Read the model definition and answer for the solid it produces. Units are mm, in the model's axes. Face numbers are marked on the shaded views. Coordinates: 2 decimals unless noted, no trailing zeros. Order: outer loops, then holes, each group sorted by start corner. A loop starts at its lowest first (then second) coordinate and runs counter-clockwise, first axis right, second up. Notation, with made-up numbers: M 20.5,1.5 L 29.5,1.5 A17 cw 29.5,17.5 Z; hole C -2,-31 d8. An arc over 180 degrees is marked long. Use a Markdown table: item, result. Add a question column.
1) Find the intervals of material crossed by probe 1 along X at (y, z) = (145, 0); probe 2 along X at (y, z) = (59.5, -2), in increasing order. Write a range as [from, to].
2) The mould has two halves that part along Y. Classify the marked faces 1 and 2: released by +Y, released by -Y, zero draft, split by the parting line, or undercut.
3) Each of these flat-tipped pins is pushed along its axis until it touches: pin 1 Ø8 at (y, z) = (69, 6) entering from +X; pin 2 Ø3.5 at (x, y) = (-145, 145) entering from +Z; pin 3 Ø10 at (x, y) = (65, 15.5) entering from +Z; pin 4 Ø8 at (x, y) = (68.5, -74) entering from -Z. Where does it stop, or does it pass through?
4) Find section A-A on x = 79. Write down the section's boundary in (y, z), plus the area to 3 significant figures.
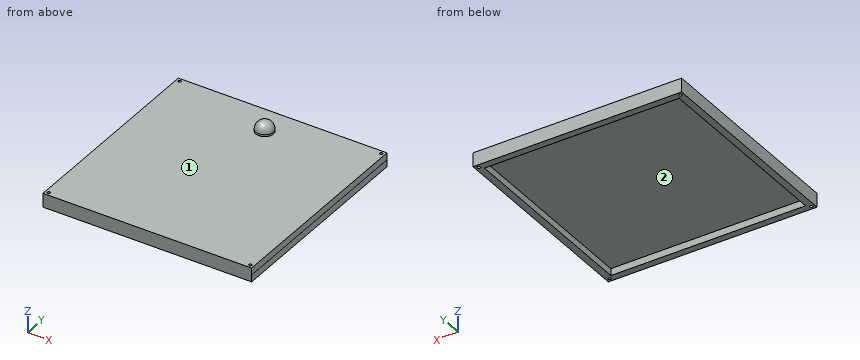
Autodesk Inventor part; units mm, degrees
ref_plane "YZ Plane" through (0, 0, 0) normal (1, 0, 0) x (0, 1, 0)
ref_plane "XZ Plane" through (0, 0, 0) normal (0, 1, 0) x (-1, 0, 0)
ref_plane "XY Plane" through (0, 0, 0) normal (0, 0, 1) x (1, 0, 0)
sketch "Sketch1" plane through (0, 0, 0) normal (0, 0, 1) x (1, 0, 0)
  line L0 (-150, 150) -> (150, 150)
  line L1 (150, 150) -> (150, -150)
  line L2 (150, -150) -> (-150, -150)
  line L3 (-150, -150) -> (-150, 150)
  point P0 (0, 0)
  point P1 (0, 150)
  point P2 (150, 0)
  dimension "d0" = 300
  dimension "d1" = 300
extrude "Extrusion1" add sketch "Sketch1" along normal blind 10
sketch "Sketch2" plane through (0, 0, 0) normal (0, 0, -1) x (-1, 0, 0)
  line L0 (150, -150) -> (-150.0258, -150)
  line L1 (-150.0258, -150) -> (-150.0258, 150)
  line L2 (-150.0258, 150) -> (150, 150)
  line L3 (150, 150) -> (150, -150)
  line L4 (-140.0258, -140) -> (140, -140)
  line L5 (140, -140) -> (140, 140)
  line L6 (140, 140) -> (-140.0258, 140)
  line L7 (-140.0258, 140) -> (-140.0258, -140)
  point P0 (0, 0)
  dimension "d4" = 10
extrude "Extrusion2" add sketch "Sketch2" along normal blind 10
sketch "Sketch3" plane through (0, 0, 10) normal (0, 0, 1) x (1, 0, 0)
  circle A0 centre (-145, 145) radius 2.05
  circle A1 centre (145, 145) radius 2.05
  line L0 (-145, 145) -> (145, 145) construction
  line L1 (150, 150) -> (-150, 150) construction
  line L2 (-150, 150) -> (-150, -150) construction
  point P0 (0, 0)
  point P1 (0, 145)
  point P2 (0, 150)
  dimension "d7" = 5
  dimension "d8" = 4.1
  dimension "d9" = 4.1
  dimension "d10" = 5
extrude "Extrusion3" cut sketch "Sketch3" against normal up to surface (20 mm away)
mirror "Mirror1" about plane through (0, 0, 0) normal (0, 1, 0) of "Extrusion3"
sketch "Sketch4" plane through (0, 0, 10) normal (0, 0, 1) x (1, 0, 0)
  circle A0 centre (0, 110) radius 12.7
  point P0 (0, 0)
  dimension "d13" = 25.4
  dimension "d17" = 110
extrude "Extrusion4" add sketch "Sketch4" along normal blind 15
fillet "Fillet1" radius 12.25 1 edges at (-12.7, 110, 25)
properties part number "locomotion top"
Check result:
| question | item | result |
|---|---|---|
| 1 | probe 1 | x = [-150, -147.05], [-142.95, 142.95], [147.05, 150] |
| 1 | probe 2 | x = [-150, -140], [140.03, 150.03] |
| 2 | face 1 | zero draft |
| 2 | face 2 | undercut |
| 3 | pin 1 | stops at x = 150 |
| 3 | pin 2 | passes through |
| 3 | pin 3 | stops at z = 10 |
| 3 | pin 4 | stops at z = 0 |
| 4 | outline | M -150,-10 L -140,-10 L -140,0 L 140,0 L 140,-10 L 150,-10 L 150,10 L -150,10 Z |
| 4 | area | 3,200 mm2 |
